Source: CAD feature listing. Evaluate the final solid. Frame: model axes, mm. Face numbers are marked on the shaded views. A direction names the side the tool comes from. Coordinates: 2 decimals unless noted, no trailing zeros. Write each loop counter-clockwise with the first axis right and the second up, starting at its lowest first coordinate (ties: lowest second). Pieces come first, ordered by that corner, then holes. Notation, with made-up numbers: (-39.75, 61) - (5.25, 61) arc R10 cw to (5.25, 74) - close; hole circle Ø7 at (74.25, -21.5). An arc over 180 degrees is marked (long way). One line per item, written item: value.
from build123d import *

# Parameters (mm, degrees)
BOSS_EXTRUDE1_DEPTH = 82.5
SKETCH3_W           = 10
SKETCH3_H           = 165
BOSS_EXTRUDE2_DEPTH = 20


with BuildPart() as part:
    # Sketch2 → Boss-Extrude1 (new body, symmetric)
    with BuildSketch(Plane.XY):
        with BuildLine():
            Line((-55, 0), (-45, 0))
            ThreePointArc((-45, 0), (0, 45), (45, 0))
            Line((45, 0), (55, 0))
            ThreePointArc((55, 0), (0, 55), (-55, 0))
        make_face()
    extrude(amount=BOSS_EXTRUDE1_DEPTH, both=True)

    # Sketch3 → Boss-Extrude2 (add)
    with BuildSketch(Plane.XZ):
        with Locations((50, 0)):
            Rectangle(SKETCH3_W, SKETCH3_H)
    extrude(amount=BOSS_EXTRUDE2_DEPTH)


solid = part.part
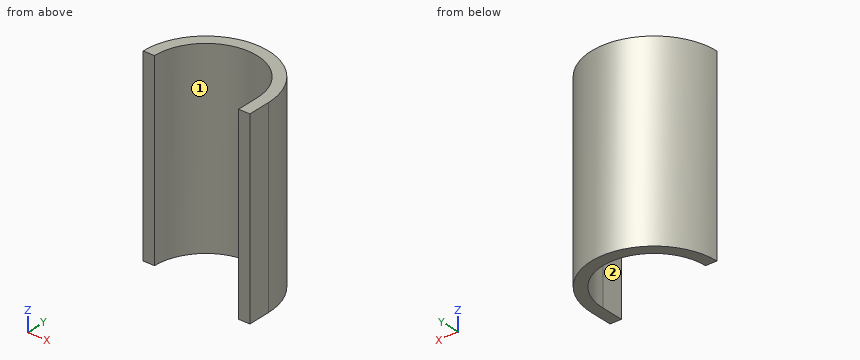
1) Material intervals for line 1 (X direction, y = 31.5, z = 33); line 2 (X direction, y = -2, z = -12.5); line 3 (X direction, y = 24, z = 14), sorted ascending.
Values found:
line 1: -45.09 to -32.14, 32.14 to 45.09
line 2: 45 to 55
line 3: -49.49 to -38.07, 38.07 to 49.49
2) Reachability of the marked faces 1 and 2 from +Z, -Z, +X, -X, +Y, -Y: full face, straight path, thin tool, end or side. Return the list, or none.
Values found:
face 1: +Z, -Z, -Y
face 2: +Z, -Z, -X, -Y
3) Section query B-B on z = -56.5. Output: boundary loops of the cut face in (x, y).
Values found:
outline: (-55, 0) - (-45, 0) arc R45 cw to (45, 0) - (45, -20) - (55, -20) - (55, 0) arc R55 ccw to start
4) Contact query for flat-ended pins moving along their axis: P1, Ø1.5, axis at x = -31.5, z = 54.5, coming from the +Y side; P2, Ø5, axis at x = 9, z = 61.5, coming from the -Y side; P3, Ø22, axis at y = -8.5, z = -17, coming from the -X side; P4, Ø8, axis at x = -51.5, z = -33.5, coming from the -Y side. Output: stop coordinate, or through.
Values found:
P1: y = 45.6
P2: y = 43.51
P3: x = -55
P4: y = 0
5) Section query C-C on x = 0. Output: boundary loops of the cut face in (y, z).
Values found:
outline: (45, -82.5) - (55, -82.5) - (55, 82.5) - (45, 82.5) - close
6) Section query A-A on y = 22.5. Output: boundary loops of the cut face in (x, z).
Values found:
outline: (-50.19, -82.5) - (-38.97, -82.5) - (-38.97, 82.5) - (-50.19, 82.5) - close; (38.97, -82.5) - (50.19, -82.5) - (50.19, 82.5) - (38.97, 82.5) - close
